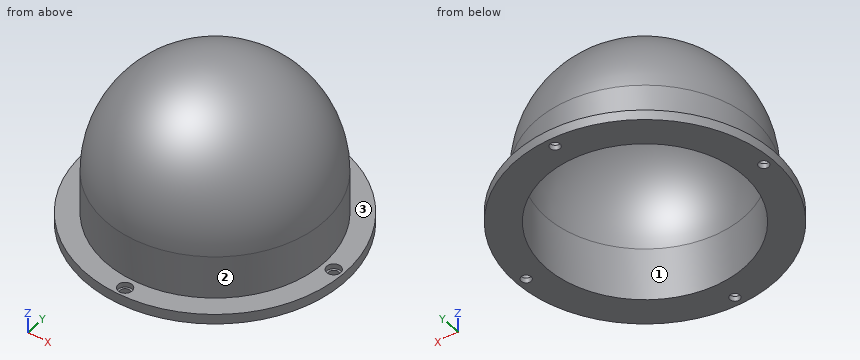
```python
from build123d import *

# Parameters (mm, degrees)
SKETCH2_R           = 65
BOSS_EXTRUDE1_DEPTH = 5
SKETCH3_R           = 54.61
BOSS_EXTRUDE2_DEPTH = 76.2
FILLET8_R           = 54.61
SKETCH7_R           = 2.5
CUT_EXTRUDE2_DEPTH  = 5
SKETCH8_R           = 3.5
CUT_EXTRUDE3_DEPTH  = 2.5
CIRPATTERN1_COUNT   = 4


# Read off the part's stored shape, not the designer's step: Shell1
with BuildPart() as part:
    # Sketch2 → Boss-Extrude1 (new body)
    with BuildSketch(Plane(origin=(0, 0, 0), x_dir=(0, 1, 0), z_dir=(0, 0, 1))):
        with Locations(Location((0, 0, 0), (0, 0, 270))):
            Circle(SKETCH2_R)
    extrude(amount=BOSS_EXTRUDE1_DEPTH)

    # Sketch3 → Boss-Extrude2 (add)
    with BuildSketch(Plane.XY.offset(5)):
        with Locations(Location((0, 0, 0), (0, 0, 180))):
            Circle(SKETCH3_R)
    extrude(amount=BOSS_EXTRUDE2_DEPTH)

    # Fillet8
    fillet8_edges = [part.edges().sort_by_distance(p)[0] for p in [
        (54.61, 0, 81.2),
    ]]
    fillet(fillet8_edges, radius=FILLET8_R)

    # Shell1 outline → Shell1 (revolve, cut)
    with BuildSketch(Plane.XZ):
        with BuildLine():
            Line((49.61, 0), (49.61, 26.58999995))
            ThreePointArc((49.61, 26.58999995), (35.079567432, 61.669567397), (0, 76.2))
            Line((0, 76.2), (0, 0))
            Line((0, 0), (49.61, 0))
        make_face()
    revolve(axis=Axis((0, 0, 0), (0, 0, 1)), mode=Mode.SUBTRACT)

    # Sketch7 → Cut-Extrude2 (cut)
    with BuildSketch(Plane.XY.offset(5)):
        with Locations((0, 60.247846794)):
            Circle(SKETCH7_R)
    cut_extrude2 = extrude(amount=-CUT_EXTRUDE2_DEPTH, mode=Mode.SUBTRACT)

    # Sketch8 → Cut-Extrude3 (cut)
    with BuildSketch(Plane.XY.offset(5)):
        with Locations((0, 60.223600104)):
            Circle(SKETCH8_R)
    cut_extrude3 = extrude(amount=-CUT_EXTRUDE3_DEPTH, mode=Mode.SUBTRACT)

    # CirPattern1: Cut-Extrude2, Cut-Extrude3 ×4 about axis
    cirpattern1_axis = Axis((0, 0, 0), (0, 0, 1))
    add([cut_extrude2.rotate(cirpattern1_axis, i * 360 / CIRPATTERN1_COUNT) for i in range(1, CIRPATTERN1_COUNT)], mode=Mode.SUBTRACT)
    add([cut_extrude3.rotate(cirpattern1_axis, i * 360 / CIRPATTERN1_COUNT) for i in range(1, CIRPATTERN1_COUNT)], mode=Mode.SUBTRACT)


solid = part.part
```
Model file for the job. Use its own axes, mm. Face numbers are marked on the shaded views. Give positions to 0.01 mm unless a question says otherwise; leave off trailing zeros. Write each loop counter-clockwise with the first axis right and the second up, starting at its lowest first coordinate (ties: lowest second). Pieces come first, ordered by that corner, then holes. Notation, with made-up numbers: (-10.5, -18) -> (12.5, -18) arc R23 ccw to (12.5, 21) -> close; hole circle Ø11 at (64, 40.25). An arc over 180 degrees is marked (long way). Use CSV: the item, a comma, the result in double quotes. Start each with the question number.
1) Cut at A-A on x = 0. List the corners of the cut face in (y, z).
2) Two-plate mould, pull along X, no slides. Class the marked faces 1, 2 and 3: released by +X, released by -X, zero draft, split by the parting line, or undercut.
3) Drill centre lines: L1, parallel to Y at x = 0, z = 4.3; L2, parallel to Y at x = 0, z = 20.25; L3, parallel to Y at x = -35, z = 34.5. Where is each one in solid material? Low to high.
4) Cut at C-C on x = 46.5. List the corners of the cut face in (y, z).
5) Cut at D-D on y = 43. List the corners of the cut face in (x, z).
6) Pin check, flat tips, straight feed: P1, Ø3, axis at x = 60.25, y = 0, coming from the +Z side; P2, Ø8, axis at x = 0, y = 60.25, coming from the +Z side; P3, Ø5.5, axis at x = 0, y = 60.22, coming from the +Z side; P4, Ø3, axis at y = -51, z = 10, coming from the +X side. Stop position of each tip, or through.
Final values:
1,outline,"(-65, 0) -> (-62.75, 0) -> (-62.75, 2.5) -> (-63.72, 2.5) -> (-63.72, 5) -> (-65, 5) -> close; (-57.75, 0) -> (-49.61, 0) -> (-49.61, 26.59) arc R49.61 cw to (49.61, 26.59) -> (49.61, 0) -> (57.75, 0) -> (57.75, 2.5) -> (56.72, 2.5) -> (56.72, 5) -> (54.61, 5) -> (54.61, 26.59) arc R54.61 ccw to (-54.61, 26.59) -> (-54.61, 5) -> (-56.72, 5) -> (-56.72, 2.5) -> (-57.75, 2.5) -> close; (62.75, 0) -> (65, 0) -> (65, 5) -> (63.72, 5) -> (63.72, 2.5) -> (62.75, 2.5) -> close"
2,face 1,"undercut"
2,face 2,"split by the parting line"
2,face 3,"zero draft"
3,L1,"y = -65 to -63.72, -56.72 to -49.61, 49.61 to 56.72, 63.72 to 65"
3,L2,"y = -54.61 to -49.61, 49.61 to 54.61"
3,L3,"y = -41.17 to -34.26, 34.26 to 41.17"
4,outline,"(-45.42, 0) -> (-17.29, 0) -> (-17.29, 26.59) arc R17.29 cw to (17.29, 26.59) -> (17.29, 0) -> (45.42, 0) -> (45.42, 5) -> (28.64, 5) -> (28.64, 26.59) arc R28.64 ccw to (-28.64, 26.59) -> (-28.64, 5) -> (-45.42, 5) -> close"
5,outline,"(-48.74, 0) -> (-24.74, 0) -> (-24.74, 26.59) arc R24.74 cw to (24.74, 26.59) -> (24.74, 0) -> (48.74, 0) -> (48.74, 5) -> (33.66, 5) -> (33.66, 26.59) arc R33.66 ccw to (-33.66, 26.59) -> (-33.66, 5) -> (-48.74, 5) -> close"
6,P1,"passes through"
6,P2,"stops at z = 5"
6,P3,"stops at z = 2.5"
6,P4,"stops at x = 23.07"
